Autodesk Inventor part; units mm, degrees
ref_plane "Plan YZ" through (0, 0, 0) normal (1, 0, 0) x (0, 1, 0)
ref_plane "Plan XZ" through (0, 0, 0) normal (0, 1, 0) x (-1, 0, 0)
ref_plane "Plan XY" through (0, 0, 0) normal (0, 0, 1) x (1, 0, 0)
sketch "Esquisse1" plane through (0, 0, 0) normal (0, 0, 1) x (1, 0, 0)
  arc A0 (-3.575, 1.45) -> (-3.575, -1.45) centre (-5.025, 0) ccw
  line L0 (-5.025, 0) -> (-3.575, -1.45) construction
  line L1 (-5.025, 0) -> (-2.9744, 0) construction
  line L2 (-5.025, 0) -> (-3.575, 1.45) construction
  line L3 (-3.575, 1.45) -> (0, 1.45)
  line L4 (-3.575, -1.45) -> (0, -1.45)
  line L5 (0, -2.8709) -> (0, 2.8709) construction
  arc A1 (3.575, -1.45) -> (3.575, 1.45) centre (5.025, 0) ccw
  line L6 (3.575, 1.45) -> (0, 1.45)
  line L7 (3.575, -1.45) -> (0, -1.45)
  line L8 (-9.9059, 0) -> (9.9059, 0) construction
  point P0 (0, 0)
  dimension "d0" = 45
  dimension "d1" = 90
  dimension "d2" = 2.9
  dimension "d3" = 5.025
extrude "Extrusion1" add sketch "Esquisse1" along normal blind 3
fillet "Congé1" radius 0.9 4 edges at (-3.575, -1.45, 1.5) (3.575, -1.45, 1.5) (3.575, 1.45, 1.5) (-3.575, 1.45, 1.5)
properties part number "T2601_Conn" material "."
Check sheet for the modelled part. Datum: model origin and axes. Units: mm. A direction names the side the tool comes from. Round coordinates to 2 decimals unless told otherwise and drop trailing zeros. Loops run counter-clockwise (first coordinate to the right, second up) from the corner with the lowest first, then second, coordinate; pieces in that order, holes last. Notation, with made-up numbers: (63, -23) -> (106, -23) arc R31 cw to (106, 2) -> close; hole circle Ø11 at (50.5, 25). An arc over 180 degrees is marked (long way). Put each result on its own line as item: value. Start each with the question number.
1. Draft check along X on faces 1 (the face through (0, 1.45, 1)), 2 (the face through (0, 0, 0)), 3 (the face through (7.075, 0.064, 1.479)). Enter one of: +X half, -X half, draft (parallel to the pull), parting line (faces both ways), or undercut.
2. Section check B-B (x = 0.5). Enter the section's corners in (y, z), plus the area to 3 significant figures.
3. Scan lines: probe 1 along X at (y, z) = (-1.7, 1.6); probe 2 along Y at (x, z) = (1.25, 0.65); probe 3 along X at (y, z) = (1.6, 2.95). Record each from-to range of solid material in increasing order.
4. Section check A-A (z = 2.2). Enter the section's corners in (x, y) (3 decimals), plus the area to 3 significant figures.
5. Gauge pin test, flat end, axial feed: pin 1 (1.5 mm diameter, centred on x = -2, z = 1.5, fed in from -Y). Record the tip position at first contact, or that the pin passes through.
6. Access from +Z, -Z, +X, -X, +Y, -Y to the whole of each face (thin tool, end or side, straight path). Record for faces 4 (the face through (0, 0, 3)), 5 (the face through (0, -1.45, 1)).
7. Section check C-C (y = 1.2). Enter the section's corners in (x, z), plus the area to 3 significant figures.
Findings:
1. face 1: undercut
1. face 2: draft
1. face 3: undercut
2. outline: (-1.45, 0) -> (1.45, 0) -> (1.45, 3) -> (-1.45, 3) -> close
2. area: 8.70 mm^2
3. probe 1: x = -6.17 to -3.88, 3.88 to 6.17
3. probe 2: y = -1.45 to 1.45
3. probe 3: x = -6.31 to -3.74, 3.74 to 6.31
4. outline: (-3.785, -1.633) arc R0.9 cw to (-3.241, -1.45) -> (3.241, -1.45) arc R0.9 cw to (3.785, -1.633) arc R2.051 ccw (long way) to (3.785, 1.633) arc R0.9 cw to (3.241, 1.45) -> (-3.241, 1.45) arc R0.9 cw to (-3.785, 1.633) arc R2.051 ccw (long way) to start
4. area: 44.8 mm^2
5. pin 1: stops at y = -1.45
6. face 4: +Z, +X, -X, +Y, -Y
6. face 5: +Z, -Z, -Y
7. outline: (-6.69, 0) -> (6.69, 0) -> (6.69, 3) -> (-6.69, 3) -> close
7. area: 40.1 mm^2
